Geometry check sheet. Reference: the model listing, model coordinates, mm. A direction names the side the tool comes from. Round coordinates to 2 decimals unless told otherwise and drop trailing zeros. Write each loop counter-clockwise with the first axis right and the second up, starting at its lowest first coordinate (ties: lowest second). Pieces come first, ordered by that corner, then holes.
Item 1: Cross-section at A-A (x = -36.9). Enter the section's corners in (y, z).
Item 2: Depth check by flat-ended pin: P1, Ø3.5, axis at x = -36.9, z = 18.73, coming from the -Y side; P2, Ø2, axis at x = 2, z = 25.5, coming from the +Y side; P3, Ø2.5, axis at x = 48.5, z = 0.5, coming from the +Y side. Enter the tip coordinate at first touch or a pass-through.
Item 3: Scan lines: probe 1 along Z at (x, y) = (-31, 64.5); probe 2 along X at (y, z) = (31, 32.5); probe 3 along Y at (x, z) = (8.5, 31). Record each from-to range of solid material in increasing order.
Item 4: Access from +Z, -Z, +X, -X, +Y, -Y to the whole of each face (thin tool, end or side, straight path). Record for faces 4 (the face through (50, 35, 1)), 5 (the face through (-50, 35, 1)), 6 (the face through (-48, 17, 12.5)), 7 (the face through (-1, 40, -50)), 8 (the face through (48, 61, -12.5)).
Item 5: Cross-section at C-C (z = 32.5). Enter the section's corners in (x, y).
Item 6: Cross-section at B-B (y = 28). Enter the section's corners in (x, z), then the cut area to 3 significant figures.
Item 7: Draft check along Y on faces 1 (the face through (-1, 40, 50)), 2 (the face through (-48, 71, 0)), 3 (the face through (47, 10, 0)). Enter one of: pulls with the +Y half, pulls with the -Y half, needs draft (parallel to the pull), parting line crosses it, or undercut.
from build123d import *

# Parameters (mm, degrees)
SKETCH1_W           = 100
SKETCH1_H           = 120
BOSS_EXTRUDE1_DEPTH = 10
SKETCH2_W           = 100
SKETCH2_H           = 5
CUT_EXTRUDE1_DEPTH  = 5
SKETCH3_R           = 2
CUT_EXTRUDE2_DEPTH  = 10
SKETCH4_W           = 100
SKETCH4_H           = 120
SKETCH4_W_2         = 90
SKETCH4_H_2         = 100
BOSS_EXTRUDE2_DEPTH = 61
SKETCH5_W           = 25
SKETCH5_H           = 15
CUT_EXTRUDE3_DEPTH  = 29
SKETCH6_W           = 25
SKETCH6_H           = 20
CUT_EXTRUDE4_DEPTH  = 29


with BuildPart() as part:
    # Sketch1 → Boss-Extrude1 (new body)
    with BuildSketch(Plane(origin=(0, 0, 0), x_dir=(1, 0, 0), z_dir=(0, 1, 0))):
        Rectangle(SKETCH1_W, SKETCH1_H)
    extrude(amount=BOSS_EXTRUDE1_DEPTH)

    # Sketch2 → Cut-Extrude1 (cut)
    with BuildSketch(Plane(origin=(0, 10, 0), x_dir=(1, 0, 0), z_dir=(0, 1, 0))):
        Rectangle(SKETCH2_W, SKETCH2_H)
    extrude(amount=-CUT_EXTRUDE1_DEPTH, mode=Mode.SUBTRACT)

    # Sketch3 → Cut-Extrude2 (cut)
    with BuildSketch(Plane(origin=(0, 10, 0), x_dir=(1, 0, 0), z_dir=(0, 1, 0))):
        with Locations(Location((13.1, -18.726688176, 0), (0, 0, 270))):
            Circle(SKETCH3_R)
        with Locations(Location((-36.9, -18.726688176, 0), (0, 0, 270))):
            Circle(SKETCH3_R)
    extrude(amount=-CUT_EXTRUDE2_DEPTH, mode=Mode.SUBTRACT)

    # Sketch4 → Boss-Extrude2 (add)
    with BuildSketch(Plane(origin=(0, 10, 0), x_dir=(1, 0, 0), z_dir=(0, 1, 0))):
        Rectangle(SKETCH4_W, SKETCH4_H)
        Rectangle(SKETCH4_W_2, SKETCH4_H_2, mode=Mode.SUBTRACT)
    extrude(amount=BOSS_EXTRUDE2_DEPTH)

    # Sketch5 → Cut-Extrude3 (cut)
    with BuildSketch(Plane.ZY.offset(50)):
        with Locations((0, 17.5)):
            Rectangle(SKETCH5_W, SKETCH5_H)
    extrude(amount=-CUT_EXTRUDE3_DEPTH, mode=Mode.SUBTRACT)

    # Sketch6 → Cut-Extrude4 (cut)
    with BuildSketch(Plane(origin=(50, 0, 0), x_dir=(0, 0, -1), z_dir=(1, 0, 0))):
        with Locations((0, 61)):
            Rectangle(SKETCH6_W, SKETCH6_H)
    extrude(amount=-CUT_EXTRUDE4_DEPTH, mode=Mode.SUBTRACT)


solid = part.part
Resolved:
1. outline: (0, -60) - (71, -60) - (71, -50) - (10, -50) - (10, -2.5) - (5, -2.5) - (5, 2.5) - (10, 2.5) - (10, 16.73) - (0, 16.73) - close; (0, 20.73) - (10, 20.73) - (10, 50) - (71, 50) - (71, 60) - (0, 60) - close
2. P1: passes through
2. P2: stops at y = 10
2. P3: stops at y = 51
3. probe 1: z = -60 to -50, 50 to 60
3. probe 2: x = -50 to -45, 45 to 50
3. probe 3: y = 0 to 10
4. face 4: +Z, -Z, +X, +Y, -Y
4. face 5: +Z, -Z, -X, +Y, -Y
4. face 6: -X
4. face 7: +Y
4. face 8: +X, +Y
5. outline: (-50, 0) - (50, 0) - (50, 71) - (45, 71) - (45, 10) - (-45, 10) - (-45, 71) - (-50, 71) - close
6. outline: (-50, -60) - (50, -60) - (50, 60) - (-50, 60) - close; hole (-45, -50) - (45, -50) - (45, 50) - (-45, 50) - close
6. area: 3,000 mm2
7. face 1: needs draft
7. face 2: pulls with the +Y half
7. face 3: undercut
